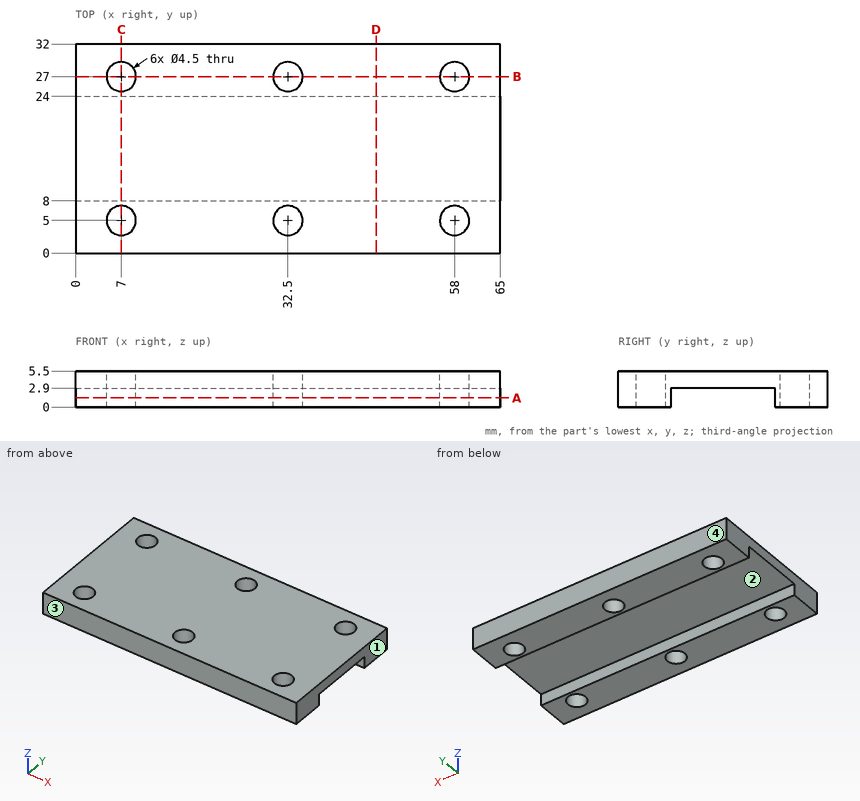
Verification items for this drawing (mm, ordinates from the low corner). Round coordinates to 2 decimals unless told otherwise and drop trailing zeros. Order: outer loops, then holes, each group sorted by start corner. A loop starts at its lowest first (then second) coordinate and runs counter-clockwise, first axis right, second up. Notation, with made-up numbers: (6.5, 7) - (40.5, 7) arc R8 cw to (40.5, 11) - close; hole circle Ø8 at (-27, 53). An arc over 180 degrees is marked (long way). Use CSV: the item, a comma, the result in double quotes.
(1) Section check A-A on z = 1.4. Record the boundary of the cut face in (x, y).
Entries:
outline,"(0, 0) - (65, 0) - (65, 8) - (0, 8) - close; (0, 24) - (65, 24) - (65, 32) - (0, 32) - close; hole circle Ø4.5 at (7, 5); hole circle Ø4.5 at (7, 27); hole circle Ø4.5 at (32.5, 5); hole circle Ø4.5 at (32.5, 27); hole circle Ø4.5 at (58, 5); hole circle Ø4.5 at (58, 27)"
(2) Section check B-B on y = 27. Record the boundary of the cut face in (x, z).
Entries:
outline,"(0, 0) - (4.75, 0) - (4.75, 5.5) - (0, 5.5) - close; (9.25, 0) - (30.25, 0) - (30.25, 5.5) - (9.25, 5.5) - close; (34.75, 0) - (55.75, 0) - (55.75, 5.5) - (34.75, 5.5) - close; (60.25, 0) - (65, 0) - (65, 5.5) - (60.25, 5.5) - close"
(3) Mould release check, pull along Y, two halves, no side actions. Record for the marked faces 1, 2, 3 and 4: released by +Y, released by -Y, zero draft, split by the parting line, or undercut.
Entries:
face 1,"zero draft"
face 2,"undercut"
face 3,"released by -Y"
face 4,"released by +Y"
(4) Section check C-C on x = 7. Record the boundary of the cut face in (y, z), and give its area (3 significant figures).
Entries:
outline,"(0, 0) - (2.75, 0) - (2.75, 5.5) - (0, 5.5) - close; (7.25, 0) - (8, 0) - (8, 2.9) - (24, 2.9) - (24, 0) - (24.75, 0) - (24.75, 5.5) - (7.25, 5.5) - close; (29.25, 0) - (32, 0) - (32, 5.5) - (29.25, 5.5) - close"
area,"80.1 mm^2"
(5) Thickness scan on probe 1 along X at (y, z) = (5, 1.8); probe 2 along Y at (x, z) = (7, 1.2); probe 3 along Y at (x, z) = (39.5, 1.85). Record the ranges inside material, lowest first. Write a range as from..to.
Entries:
probe 1,"0..4.75, 9.25..30.25, 34.75..55.75, 60.25..65"
probe 2,"0..2.75, 7.25..8, 24..24.75, 29.25..32"
probe 3,"0..8, 24..32"
(6) Section check D-D on x = 46. Record the boundary of the cut face in (y, z), and give its area (3 significant figures).
Entries:
outline,"(0, 0) - (8, 0) - (8, 2.9) - (24, 2.9) - (24, 0) - (32, 0) - (32, 5.5) - (0, 5.5) - close"
area,"130 mm^2"
(7) Gauge pin test, flat ends, axial feed: pin 1 Ø3 at (x, z) = (25, 2) entering from -Y; pin 2 Ø8 at (x, y) = (22, 16) entering from -Z. Record the tip position at first contact, or that the pin passes through.
Entries:
pin 1,"y = 0"
pin 2,"z = 2.9"
